Geometry check sheet. Reference: the model listing, model coordinates, mm. A direction names the side the tool comes from. Coordinates: 2 decimals unless noted, no trailing zeros. Write each loop counter-clockwise with the first axis right and the second up, starting at its lowest first coordinate (ties: lowest second). Pieces come first, ordered by that corner, then holes.
from build123d import *

# Parameters (mm, degrees)
BOX036_W       = 150.2
BOX036_H       = 200.2
BOX036_DEPTH   = 25
FILLET022_R    = 30
FILLET023_R    = 30
FILLET024_R    = 30
FILLET025_R    = 30
THICKNESS001_T = 2


with BuildPart() as part:
    # Box036 → Box036 (new body)
    with BuildSketch(Plane.XY):
        with Locations((75.1, 100.1)):
            Rectangle(BOX036_W, BOX036_H)
    extrude(amount=BOX036_DEPTH)

    # Fillet022
    fillet022_edges = [part.edges().sort_by_distance(p)[0] for p in [
        (150.2, 0, 12.5),
    ]]
    fillet(fillet022_edges, radius=FILLET022_R)

    # Fillet023
    fillet023_edges = [part.edges().sort_by_distance(p)[0] for p in [
        (150.2, 200.2, 12.5),
    ]]
    fillet(fillet023_edges, radius=FILLET023_R)

    # Fillet024
    fillet024_edges = [part.edges().sort_by_distance(p)[0] for p in [
        (0, 0, 12.5),
    ]]
    fillet(fillet024_edges, radius=FILLET024_R)

    # Fillet025
    fillet025_edges = [part.edges().sort_by_distance(p)[0] for p in [
        (0, 200.2, 12.5),
    ]]
    fillet(fillet025_edges, radius=FILLET025_R)

    # Thickness001
    thickness001_openings = [part.faces().sort_by_distance(p)[0] for p in [
        (75.1, 100.1, 0),
    ]]
    offset(amount=THICKNESS001_T, openings=thickness001_openings)


with BuildPart() as part_1:
    # Thickness001 placement: moved
    add(part.part.moved(Location((0, 300, 400))))


solid = part_1.part
1. Draft check along X on faces 1 (the cylindrical face through (141.645, 491.179, 412.675)), 2 (the cylindrical face through (143.07, 492.58, 412.68)), 3 (the flat face through (-2, 399, 412)). Enter one of: released by +X, released by -X, zero draft, split by the parting line, or undercut.
Computed values:
face 1: undercut
face 2: released by +X
face 3: released by -X
2. Thickness scan on line 1 along X through (y, z) = (409, 407.75); line 2 along Y through (x, z) = (71.5, 412.25); line 3 along Z through (x, y) = (22.5, 433). Record the ranges inside material, lowest first.
Computed values:
line 1: x = -2 to 0, 150.2 to 152.2
line 2: y = 298 to 300, 500.2 to 502.2
line 3: z = 425 to 427
3. Sectioned sample at A-A, the plane x = 62. Record the boundary of the cut face in (y, z).
Computed values:
outline: (298, 400) - (300, 400) - (300, 425) - (500.2, 425) - (500.2, 400) - (502.2, 400) - (502.2, 425) arc R2 ccw to (500.2, 427) - (300, 427) arc R2 ccw to (298, 425) - close
4. Sectioned sample at C-C, the plane z = 412.5. Record the boundary of the cut face in (x, y).
Computed values:
outline: (-2, 330) arc R32 ccw to (30, 298) - (120.2, 298) arc R32 ccw to (152.2, 330) - (152.2, 470.2) arc R32 ccw to (120.2, 502.2) - (30, 502.2) arc R32 ccw to (-2, 470.2) - close; hole (0, 330) arc R30 ccw to (30, 300) - (120.2, 300) arc R30 ccw to (150.2, 330) - (150.2, 470.2) arc R30 ccw to (120.2, 500.2) - (30, 500.2) arc R30 ccw to (0, 470.2) - close
5. Sectioned sample at B-B, the plane y = 408.5. Record the boundary of the cut face in (x, z).
Computed values:
outline: (-2, 400) - (0, 400) - (0, 425) - (150.2, 425) - (150.2, 400) - (152.2, 400) - (152.2, 425) arc R2 ccw to (150.2, 427) - (0, 427) arc R2 ccw to (-2, 425) - close
6. Gauge pin test, flat ends, axial feed: pin 1 Ø6 at (y, z) = (476, 421.5) entering from +X; pin 2 Ø3 at (x, y) = (115, 439.5) entering from -Z. Record the tip position at first contact, or that the pin passes through.
Computed values:
pin 1: stops at x = 152.08
pin 2: stops at z = 425
7. Access from +Z, -Z, +X, -X, +Y, -Y to the whole of each face (thin tool, end or side, straight path). Record for faces 4 (the flat face through (74, 402, 427)), 5 (the cylindrical face through (9.021, 308.555, 412.675)).
Computed values:
face 4: +Z, +X, -X, +Y, -Y
face 5: -Z
